from build123d import *

# Parameters (mm, degrees)
BOSS_EXTRUDE1_DEPTH = 25
BOSS_EXTRUDE2_DEPTH = 2.4
SKETCH3_R           = 3
SKETCH3_R_2         = 1
BOSS_EXTRUDE3_DEPTH = 2.3
BOSS_EXTRUDE4_START = 2.3
SKETCH3_3_R         = 1
BOSS_EXTRUDE4_DEPTH = 8.25
SKETCH4_R           = 28.625
BOSS_EXTRUDE5_DEPTH = 2


with BuildPart() as part:
    # Sketch1 → Boss-Extrude1 (new body)
    with BuildSketch(Plane(origin=(0, 0, 0), x_dir=(1, 0, 0), z_dir=(0, 1, 0))):
        with BuildLine():
            Line((-6.614378278, -7.5), (-6.614378278, 7.5))
            ThreePointArc((-6.614378278, 7.5), (0, 10), (6.614378278, 7.5))
            Line((6.614378278, 7.5), (6.614378278, -7.5))
            ThreePointArc((6.614378278, -7.5), (0, -10), (-6.614378278, -7.5))
        make_face()
    extrude(amount=BOSS_EXTRUDE1_DEPTH)

    # Sketch2 → Boss-Extrude2 (add)
    with BuildSketch(Plane(origin=(0, 25, 0), x_dir=(1, 0, 0), z_dir=(0, 1, 0))):
        with BuildLine():
            Line((-3.720362886, 3.25), (-3.720362886, -3.25))
            ThreePointArc((-3.720362886, -3.25), (4.94, 0), (-3.720362886, 3.25))
        make_face()
    extrude(amount=BOSS_EXTRUDE2_DEPTH)

    # Sketch3 → Boss-Extrude3 (add)
    # profile 1 of 2: a face of its own
    with BuildSketch(Plane.XZ):
        with Locations(Location((0, 0, 0), (0, 0, 270))):
            Circle(SKETCH3_R)
        Circle(SKETCH3_R_2, mode=Mode.SUBTRACT)
    # profile 2 of 2: a face of its own
    with BuildSketch(Plane.XZ):
        Circle(SKETCH3_R_2)
    extrude(amount=BOSS_EXTRUDE3_DEPTH)

    # Sketch3<3> → Boss-Extrude4 (add)
    with BuildSketch(Plane.XZ.offset(BOSS_EXTRUDE4_START)):
        with Locations(Location((0, 0, 0), (0, 0, 270))):
            Circle(SKETCH3_3_R)
    extrude(amount=BOSS_EXTRUDE4_DEPTH)

    # Sketch4 → Boss-Extrude5 (add)
    with BuildSketch(Plane(origin=(0, -10.55, 0), x_dir=(-1, 0, 0), z_dir=(0, -1, 0))):
        with Locations(Location((0, 0, 0), (0, 0, 90))):
            Circle(SKETCH4_R)
    extrude(amount=BOSS_EXTRUDE5_DEPTH)


solid = part.part
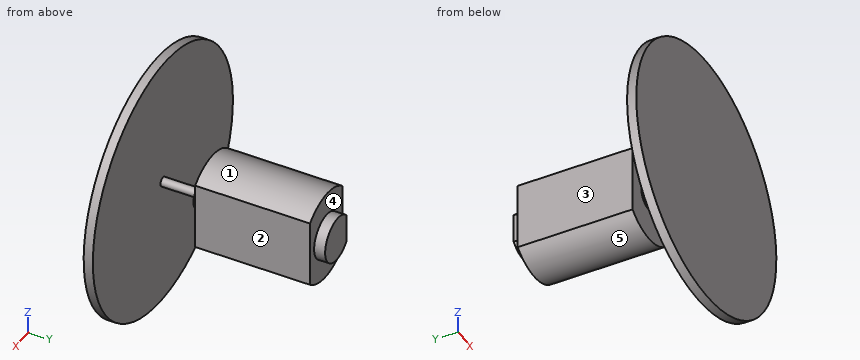
Here's how the part is built. I have some questions about the finished solid (model axes, mm). Face numbers are marked on the shaded views. A direction names the side the tool comes from. Round coordinates to 2 decimals unless told otherwise and drop trailing zeros. Loops run counter-clockwise (first coordinate to the right, second up) from the corner with the lowest first, then second, coordinate; pieces in that order, holes last.
1. For P1, Ø1.2, axis at y = 26.5, z = 0.5, coming from the -X side; P2, Ø10, axis at x = 3.5, y = 3.5, coming from the -Z side; P3, Ø4.5, axis at y = 16, z = -0.5, coming from the -X side, each with a flat end and sliding along its axis, tell me the tip position at first contact or that it passes through.
Answer list:
P1: stops at x = -3.72
P2: stops at z = -10
P3: stops at x = -6.61
2. If we section it at C-C on y = 24: Write out the boundary of the cut face in (x, z), plus the area to 3 significant figures.
Answer list:
outline: (-6.61, -7.5) arc R10 ccw to (6.61, -7.5) - (6.61, 7.5) arc R10 ccw to (-6.61, 7.5) - close
area: 244 mm2
3. If we section it at B-B on z = 0: Write out the boundary of the cut face in (x, y) (3 decimals).
Answer list:
outline: (-28.625, -12.55) - (28.625, -12.55) - (28.625, -10.55) - (1, -10.55) - (1, -2.3) - (3, -2.3) - (3, 0) - (6.614, 0) - (6.614, 25) - (4.94, 25) - (4.94, 27.4) - (-3.72, 27.4) - (-3.72, 25) - (-6.614, 25) - (-6.614, 0) - (-3, 0) - (-3, -2.3) - (-1, -2.3) - (-1, -10.55) - (-28.625, -10.55) - close
4. Which directions (+Z, -Z, +X, -X, +Y, -Y) give clear straight access to the entire face, cutting with the end or side of a thin tool? Please do the marked faces 1, 2, 3, 4 and 5.
Answer list:
face 1: +Z, +Y
face 2: +Z, -Z, +X, +Y
face 3: +Z, -Z, -X, +Y
face 4: +Y
face 5: -Z, +Y
5. If we section it at D-D on x = 21: Write out the boundary of the cut face in (y, z).
Answer list:
outline: (-12.55, -19.45) - (-10.55, -19.45) - (-10.55, 19.45) - (-12.55, 19.45) - close
6. If we section it at A-A on x = 0: Write out the boundary of the cut face in (y, z) (3 decimals), plus the area to 3 significant figures.
Answer list:
outline: (-12.55, -28.625) - (-10.55, -28.625) - (-10.55, -1) - (-2.3, -1) - (-2.3, -3) - (0, -3) - (0, -10) - (25, -10) - (25, -4.94) - (27.4, -4.94) - (27.4, 4.94) - (25, 4.94) - (25, 10) - (0, 10) - (0, 3) - (-2.3, 3) - (-2.3, 1) - (-10.55, 1) - (-10.55, 28.625) - (-12.55, 28.625) - close
area: 669 mm2
7. If I drill on line 1 along Y through (x, z) = (5.5, 5.5); line 2 along Y through (x, z) = (12, -4.5); line 3 along X through (y, z) = (1.5, 0), over which ranges is the centre line in solid material (lowest first)?
Answer list:
line 1: y = -12.55 to -10.55, 0 to 25
line 2: y = -12.55 to -10.55
line 3: x = -6.61 to 6.61
